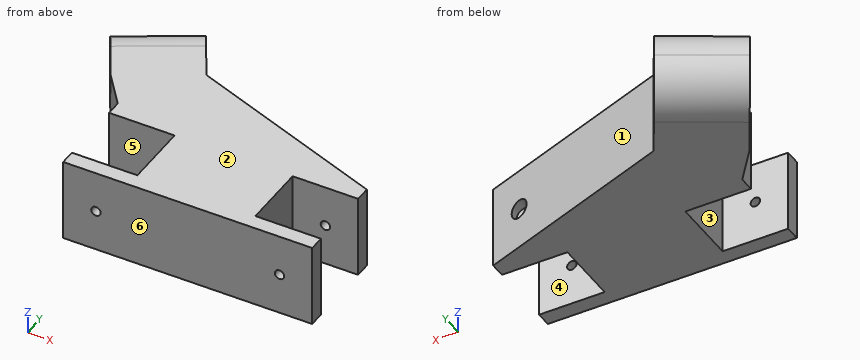
from build123d import *

# Parameters (mm, degrees)
BOSS_EXTRUDE1_DEPTH = 38.1
CUT_EXTRUDE1_DEPTH  = 84.912499942
HOLE3_D             = 25.4
HOLE4_D             = 4.300000036
HOLE4_DEPTH         = 6.99999997


with BuildPart() as part:
    # Sketch7 → Boss-Extrude1 (new body)
    with BuildSketch(Plane.XY):
        Polygon((-87.593351826, 47.625), (-54.597783942, 66.675), (-35.547783942, 33.679432116), (56.999999919, 0), (56.999999919, -6.99999997), (26.999999975, -6.99999997), (26.999999975, -36.999999914), (56.999999919, -36.999999914), (56.999999919, -43.999999884), (-56.999999919, -43.999999884), (-56.999999919, -36.999999914), (-26.999999975, -36.999999914), (-26.999999975, -6.99999997), (-56.999999919, -6.99999997), (-56.999999919, 0), (-68.543351826, 14.629432116), align=None)
    extrude(amount=BOSS_EXTRUDE1_DEPTH)

    # Sketch8 → Cut-Extrude1 (cut, through all)
    with BuildSketch(Plane(origin=(-12.077216058, -6.972783942, 0), x_dir=(0, 0, -1), z_dir=(0.866025404, 0.5, 0))):
        with BuildLine():
            ThreePointArc((-38.1, 65.991135768), (-32.520384182, 79.46151995), (-19.05, 85.041135768))
            Line((-19.05, 85.041135768), (-38.1, 85.041135768))
            Line((-38.1, 85.041135768), (-38.1, 65.991135768))
        make_face()
        with BuildLine():
            Line((0, 65.991135768), (0, 85.041135768))
            Line((0, 85.041135768), (-19.05, 85.041135768))
            ThreePointArc((-19.05, 85.041135768), (-5.579615818, 79.46151995), (0, 65.991135768))
        make_face()
    extrude(amount=-CUT_EXTRUDE1_DEPTH, mode=Mode.SUBTRACT)

    # Hole3 (through all)
    with Locations(Plane(origin=(-12.077216058, -6.972783942, 0), x_dir=(0, 0, -1), z_dir=(0.866025404, 0.5, 0))):
        with Locations((-19.05, 65.991135768)):
            Hole(HOLE3_D / 2)

    # Hole4
    with Locations(Plane.XZ.offset(43.999999884)):
        with Locations((-41.999999947, 19.05), (41.999999947, 19.05)):
            Hole(HOLE4_D / 2, depth=HOLE4_DEPTH)

    # Sketch21 → Hole5 (revolve, cut)
    with BuildSketch(Plane(origin=(41.999999947, -6.99999997, 19.05), x_dir=(0, 0, -1), z_dir=(1, 0, 0))):
        Polygon((0, 0), (0, 73.67499997), (4.300000036, 73.67499997), (4.300000036, 6.99999997), (2.150000018, 6.99999997), (2.150000018, 0), align=None)
    revolve(axis=Axis((41.999999947, 103.00000003, 19.05), (0, -1, 0)), mode=Mode.SUBTRACT)


solid = part.part
Geometry check sheet. Reference: the model listing, model coordinates, mm. Face numbers are marked on the shaded views. A direction names the side the tool comes from. Round coordinates to 2 decimals unless told otherwise and drop trailing zeros. Write each loop counter-clockwise with the first axis right and the second up, starting at its lowest first coordinate (ties: lowest second). Pieces come first, ordered by that corner, then holes. Notation, with made-up numbers: (8, 69.5) - (26, 69.5) arc R7 ccw to (26, 81.5) - close; hole circle Ø1 at (89.5, 5.25). An arc over 180 degrees is marked (long way). One line per item, written item: value.
1. Cross-section at A-A on x = 42. Record the boundary of the cut face in (y, z).
The answers:
outline: (-44, 0) - (-37, 0) - (-37, 16.9) - (-44, 16.9) - close; (-44, 21.2) - (-37, 21.2) - (-37, 38.1) - (-44, 38.1) - close; (-7, 0) - (5.46, 0) - (5.46, 14.75) - (0, 14.75) - (0, 16.9) - (-7, 16.9) - close; (-7, 21.2) - (0, 21.2) - (0, 23.35) - (5.46, 23.35) - (5.46, 38.1) - (-7, 38.1) - close
2. Set-up check for the marked faces 4, 5 and 6: record each of +Z, -Z, +X, -X, +Y, -Y from which the full face is reachable in a straight line by a thin tool's end or side.
The answers:
face 4: +Z, -Z, +X
face 5: +Z, -Z, -X
face 6: +Z, -Z, +X, -X, -Y
3. Mould release check, pull along Y, two halves, no side actions. Record for the marked faces 1, 2 and 3: released by +Y, released by -Y, zero draft, split by the parting line, or undercut.
The answers:
face 1: released by +Y
face 2: zero draft
face 3: undercut
4. Depth check by flat-ended pin: pin 1 Ø4 at (x, z) = (17, 21.5) entering from +Y; pin 2 Ø5 at (y, z) = (32.5, 23.5) entering from -X; pin 3 Ø4 at (y, z) = (54.5, 26.5) entering from -X. Enter the tip coordinate at first touch or a pass-through.
The answers:
pin 1: stops at y = 15.28
pin 2: stops at x = -56.74
pin 3: stops at x = -76.46
5. Cross-section at C-C on z = 10. Record the boundary of the cut face in (x, y), and give its area (3 significant figures).
The answers:
outline: (-86.45, 45.64) - (-82.52, 38.84) - (-49.53, 57.89) - (-53.45, 64.69) - close; (-73.61, 23.41) - (-68.54, 14.63) - (-57, 0) - (-57, -7) - (-27, -7) - (-27, -37) - (-57, -37) - (-57, -44) - (57, -44) - (57, -37) - (27, -37) - (27, -7) - (57, -7) - (57, 0) - (-35.55, 33.68) - (-40.62, 42.46) - close
area: 6,170 mm^2
6. Cross-section at B-B on y = -2.5. Record the boundary of the cut face in (x, z).
The answers:
outline: (-57, 0) - (57, 0) - (57, 38.1) - (-57, 38.1) - close; hole circle Ø4.3 at (42, 19.05)
7. Cross-section at D-D on z = 30. Record the boundary of the cut face in (x, y) (3 decimals).
The answers:
outline: (-85.863, 44.627) - (-81.285, 36.699) - (-48.289, 55.749) - (-52.867, 63.677) - close; (-74.852, 25.556) - (-68.543, 14.629) - (-57, 0) - (-57, -7) - (-27, -7) - (-27, -37) - (-57, -37) - (-57, -44) - (57, -44) - (57, -37) - (27, -37) - (27, -7) - (57, -7) - (57, 0) - (-35.548, 33.679) - (-41.856, 44.606) - close
8. Scan lines: L1, parallel to X at y = -41, z = 19; L2, parallel to Z at x = -42, y = -40.25; L3, parallel to X at y = -8.5, z = 3. Record each from-to range of solid material in increasing order.
The answers:
L1: x = -57 to -44.15, -39.85 to 39.85, 44.15 to 57
L2: z = 0 to 16.9, 21.2 to 38.1
L3: x = -27 to 27
